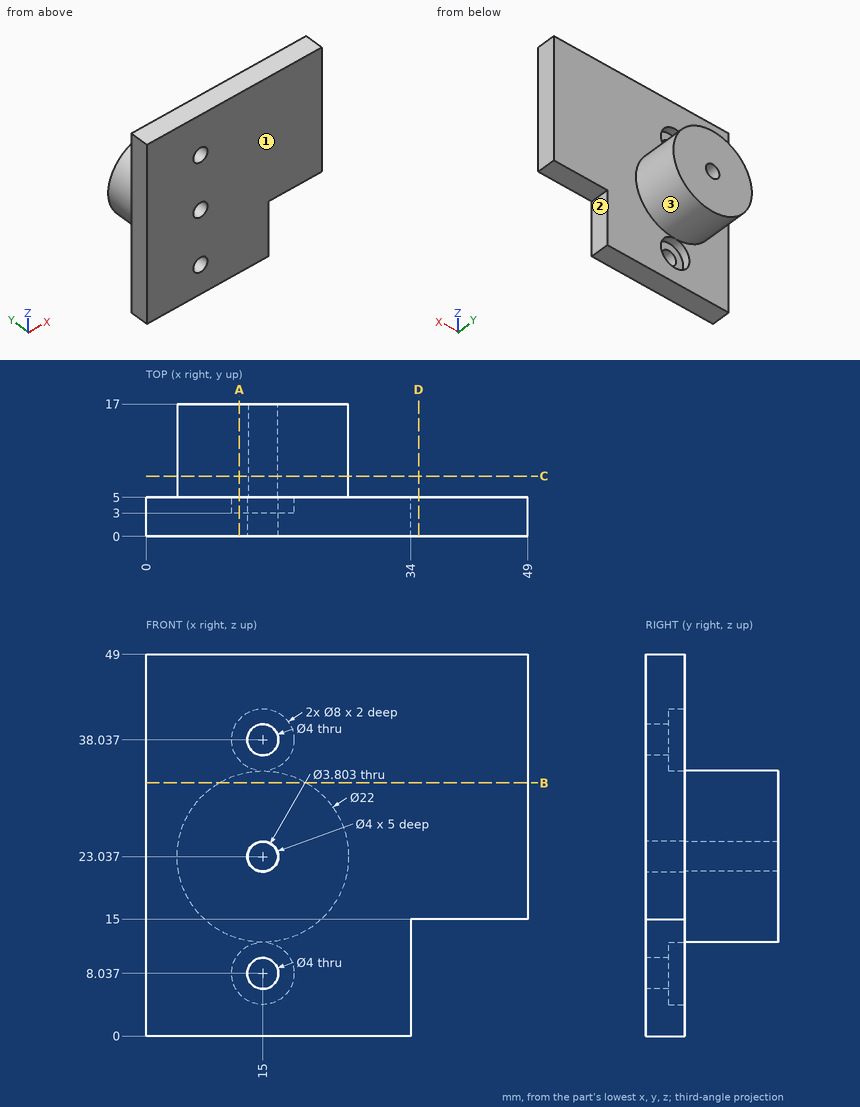
Drawing for the job (mm, zero at the part's lowest x, y, z). A direction names the side the tool comes from. Round coordinates to 2 decimals unless told otherwise and drop trailing zeros. Write each loop counter-clockwise with the first axis right and the second up, starting at its lowest first coordinate (ties: lowest second). Pieces come first, ordered by that corner, then holes. Notation, with made-up numbers: M 82,-35 L 99,-35 A6 cw 99,-30 Z; hole C 32.5,-5 d2. An arc over 180 degrees is marked long. Put each result on its own line as item: value.
Item 1: Cut at C-C (y = 7.75). List the corners of the cut face in (x, z).
Responses:
outline: C 15,23.04 d22; hole C 15,23.04 d3.8
Item 2: Tool access for the marked faces 1, 2 and 3: list every direction of +Z, -Z, +X, -X, +Y, -Y with a clear straight run to the whole face (end or side of a thin tool).
Responses:
face 1: +Z, -Z, +X, -X, -Y
face 2: -Z, +X, +Y, -Y
face 3: +Y
Item 3: Cut at A-A (x = 12). List the corners of the cut face in (y, z).
Responses:
outline: M 0,0 L 5,0 L 5,5.39 L 3,5.39 L 3,10.68 L 5,10.68 L 5,12.45 L 17,12.45 L 17,33.62 L 5,33.62 L 5,35.39 L 3,35.39 L 3,40.68 L 5,40.68 L 5,49 L 0,49 Z
Item 4: Probe L1, parallel to Z at x = 15, y = 3.8; L2, parallel to Y at x = 34, z = 40; L3, parallel to Z at x = 15.5, y = 13 (1 decimal). List the from-to ranges inside material, lowest first. Write a range as from..to.
Responses:
L1: 0..4.04, 12.04..21.04, 25.04..34.04, 42.04..49
L2: 0..5
L3: 12..21.2, 24.9..34
Item 5: Cut at B-B (z = 32.5). List the corners of the cut face in (x, y).
Responses:
outline: M 0,0 L 49,0 L 49,5 L 20.61,5 L 20.61,17 L 9.39,17 L 9.39,5 L 0,5 Z
Item 6: Cut at D-D (x = 35). List the corners of the cut face in (y, z), and give its area (3 significant figures).
Responses:
outline: M 0,15 L 5,15 L 5,49 L 0,49 Z
area: 170 mm²
Item 7: Flat gauge pins, fed straight in: P1, Ø5, axis at x = 15, z = 8.04, coming from the +Y side; P2, Ø4, axis at y = 3.5, z = 7, coming from the +X side; P3, Ø1, axis at x = 20, y = 10, coming from the +Z side (1 decimal); P4, Ø3.5, axis at x = 15, z = 38.04, coming from the -Y side. Where does each tip first touch, or does it go through?
Responses:
P1: y = 3
P2: x = 34
P3: z = 33.1
P4: through
